Design review of the part built by this model. Coordinates are the model's own, in mm. A direction names the side the tool comes from. Coordinates: 2 decimals unless noted, no trailing zeros. Write each loop counter-clockwise with the first axis right and the second up, starting at its lowest first coordinate (ties: lowest second). Pieces come first, ordered by that corner, then holes.
Q1. Take a section at A-A (y = -5.5). State how many separate pieces and enclosed holes the cut face has, and give its area (3 significant figures).
Q2. Take a section at D-D (y = -11). Give the boundary of the cut face in (x, z).
Q3. Take a section at B-B (z = -3.5). Give the boundary of the cut face in (x, y).
Q4. Take a section at C-C (x = 25). Give the boundary of the cut face in (y, z).
Q5. Mouldability with a two-part tool opening along Z and no side actions: class faces 1 (the cylindrical face through (-49.43, -11.4, 0.8)), 2 (the cylindrical face through (0.67, -0.6, -14.43)), 3 (the flat face through (-44, -6, 11.4)) as pulls with the +Z half, pulls with the -Z half, needs draft (parallel to the pull), parting line crosses it, or undercut.
Q6. Machinability: for faces 4 (the cylindrical face through (49.43, -0.6, 1.2)), 5 (the flat face through (-43, -6, 9.6)), which of the approach directions +Z, -Z, +X, -X, +Y, -Y give a long, thin tool a straight path to every point of the face, cutting with its end or side? Answer none if there is none.
Q7. For probe 1 along Z at (x, y) = (-40, -7); probe 2 along Z at (x, y) = (41.5, -4); probe 3 along X at (y, z) = (-1.5, -6.25), list the stretches that pass through material, from the lowest coordinate up.
Q8. Insertion check: pin 1 (2 mm diameter, centred on x = -40, y = -5.5, fed in from +Z); pin 2 (11.5 mm diameter, centred on x = 25, z = -5, fed in from +Y); pin 3 (1 mm diameter, centred on x = 19, y = -9, fed in from +Z). Each pin has a flat end and moves straight along its axis. Give the tip position at first contact, or say it passes through.
```python
from build123d import *

# Parameters (mm, degrees)
F1_DEPTH = 12
F2_R     = 2
F3_R     = 5
F3_R_2   = 2.5
F4_DEPTH = 12.001
F5_W     = 7
F5_H     = 1.2
F6_DEPTH = 100.001


with BuildPart() as f1:
    # F0 (on Front) → F1 (new body)
    with BuildSketch(Plane.XZ):
        with BuildLine():
            Line((-50, -15), (50, -15))
            Line((50, -15), (50, 15))
            Line((50, 15), (43.30127, 15))
            ThreePointArc((43.30127, 15), (22.912878, 3.856217), (0, 0))
            ThreePointArc((0, 0), (-22.912878, 3.856217), (-43.30127, 15))
            Line((-43.30127, 15), (-50, 15))
            Line((-50, 15), (-50, -15))
        make_face()
    extrude(amount=F1_DEPTH)

    # F2
    f2_edges = [f1.edges().sort_by_distance(p)[0] for p in [
        (0, -12, -15),
        (-50, -12, 0),
        (50, -12, 0),
        (50, 0, 0),
        (0, 0, -15),
        (-50, 0, 0),
        (-50, -6, -15),
        (50, -6, -15),
        (50, -6, 15),
        (-50, -6, 15),
    ]]
    fillet(f2_edges, radius=F2_R)

    # F3 (on face) → F4 (cut, through all)
    with BuildSketch(Plane.XZ.offset(12)):
        with Locations((-25, -5)):
            Circle(F3_R)
        with Locations((-40, 0)):
            Circle(F3_R)
        with Locations((0, -7)):
            Circle(F3_R_2)
        with Locations((25, -5)):
            Circle(F3_R)
        with Locations((40, 0)):
            Circle(F3_R)
    extrude(amount=-F4_DEPTH, mode=Mode.SUBTRACT)

    # F5 (on face) → F6 (cut, through all)
    with BuildSketch(Plane(origin=(-50, 0, 0), x_dir=(0, -1, 0), z_dir=(-1, 0, 0))):
        with Locations((6, 12)):
            Rectangle(F5_W, F5_H)
        with Locations((6, 9)):
            Rectangle(F5_W, F5_H)
    extrude(amount=-F6_DEPTH, mode=Mode.SUBTRACT)


solid = f1.part
```
Response:
1. separate pieces: 5
1. enclosed holes: 5
1. area: 1,710 mm2
2. outline: (-49.73, -13) arc R1.73 ccw to (-48, -14.73) - (48, -14.73) arc R1.73 ccw to (49.73, -13) - (49.73, 14) arc R2 ccw to (48, 15) - (43.3, 15) arc R70 cw to (0, 0) arc R70 cw to (-43.3, 15) - (-48, 15) arc R2 ccw to (-49.73, 14) - close; hole circle Ø10 at (-40, 0); hole circle Ø10 at (-25, -5); hole circle Ø5 at (0, -7); hole circle Ø10 at (25, -5); hole circle Ø10 at (40, 0)
3. outline: (-50, -10) arc R2 ccw to (-48, -12) - (-43.57, -12) - (-43.57, 0) - (-48, 0) arc R2 ccw to (-50, -2) - close; (-36.43, -12) - (-29.77, -12) - (-29.77, 0) - (-36.43, 0) - close; (-20.23, -12) - (20.23, -12) - (20.23, 0) - (-20.23, 0) - close; (29.77, -12) - (36.43, -12) - (36.43, 0) - (29.77, 0) - close; (43.57, -12) - (48, -12) arc R2 ccw to (50, -10) - (50, -2) arc R2 ccw to (48, 0) - (43.57, 0) - close
4. outline: (-12, -13) arc R2 ccw to (-10, -15) - (-2, -15) arc R2 ccw to (0, -13) - (0, -10) - (-12, -10) - close; (-12, 0) - (0, 0) - (0, 4.62) - (-12, 4.62) - close
5. face 1: needs draft
5. face 2: pulls with the -Z half
5. face 3: undercut
6. face 4: +Z, -Z, +X, +Y
6. face 5: +X, -X
7. probe 1: z = -15 to -5, 5 to 8.4, 9.6 to 11.4
7. probe 2: z = -15 to -4.77, 4.77 to 8.4, 9.6 to 11.4, 12.6 to 13.63
7. probe 3: x = -49.94 to -29.84, -20.16 to -2.38, 2.38 to 20.16, 29.84 to 49.94
8. pin 1: stops at z = 13.26
8. pin 2: stops at y = 0
8. pin 3: stops at z = 2.77
